Source: three-view drawing plus pictorial views. Frame: mm from the lowest corner of the part. A direction names the side the tool comes from. Coordinates: 2 decimals unless noted, no trailing zeros. Write each loop counter-clockwise with the first axis right and the second up, starting at its lowest first coordinate (ties: lowest second). Pieces come first, ordered by that corner, then holes. Notation, with made-up numbers: (-4.5, -16.75) - (33.5, -16.75) arc R16 cw to (33.5, -6.75) - close; hole circle Ø9 at (-21.5, 73). An arc over 180 degrees is marked (long way). Put each result on its own line as item: value. Start each with the question number.
1. Access query for the marked faces 1 and 2. Directions: +Z, -Z, +X, -X, +Y, -Y. A direction counts if a zero-diameter tool reaches every point of the face in a straight line with its end or side. Return the directions, or none.
2. Line query: line 1 (Y direction, x = 32.5, z = 78); line 2 (Y direction, x = 116.5, z = 106); line 3 (X direction, y = 51, z = 143). Output: solid intervals per line, ascending.
3. Cut plane C-C, the plane y = 25. Return loops of the section in (x, z).
4. Pin query (flat end, axial travel): pin 1 (1 mm diameter, centred on y = 60, z = 62, fed in from +X). Return the tip coordinate at first contact, or that it passes through.
5. Cut plane A-A, the plane x = 33. Return loops of the section in (y, z), and give its area (3 significant figures).
6. Cut plane B-B, the plane z = 52. Return loops of the section in (x, y), and give its area (3 significant figures).
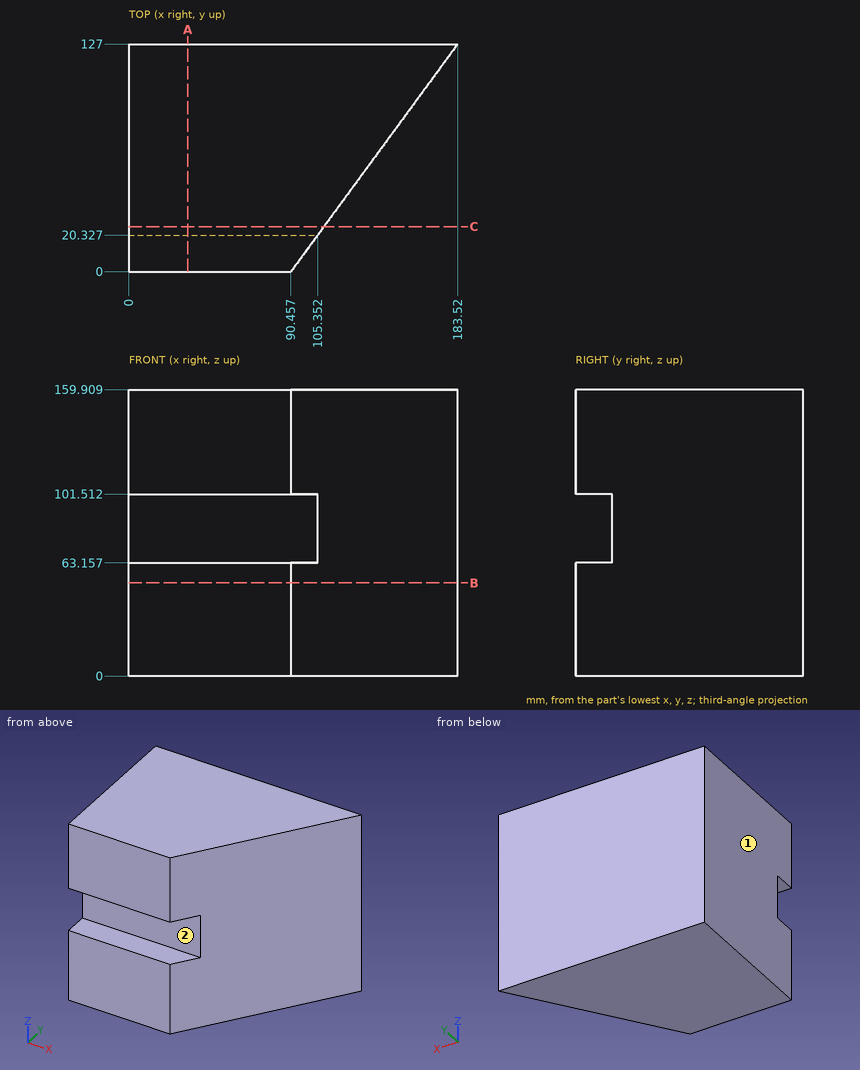
Report:
1. face 1: +Z, -Z, -X, +Y, -Y
1. face 2: +X, -X, -Y
2. line 1: y = 20.33 to 127
2. line 2: y = 35.54 to 127
2. line 3: x = 0 to 127.83
3. outline: (0, 0) - (108.78, 0) - (108.78, 159.91) - (0, 159.91) - close
4. pin 1: stops at x = 134.79
5. outline: (0, 0) - (127, 0) - (127, 159.91) - (0, 159.91) - (0, 101.51) - (20.33, 101.51) - (20.33, 63.16) - (0, 63.16) - close
5. area: 19,500 mm^2
6. outline: (0, 0) - (90.46, 0) - (183.52, 127) - (0, 127) - close
6. area: 17,400 mm^2
